from build123d import *

# Parameters (mm, degrees)
CORNER_DEPTH = 6
SKETCH2_W    = 6
SKETCH2_H    = 70
SKETCH2_H_2  = 260
MOUNT_DEPTH  = 10
FILLET1_R    = 1
LITE_DEPTH   = 391.911754748


with BuildPart() as part:
    # Sketch1 → corner (new body)
    with BuildSketch(Plane(origin=(0, 0, 0), x_dir=(0, 0, -1), z_dir=(1, 0, 0))):
        Polygon((0, 0), (0, 370), (26, 370), (126, 20), (126, 0), align=None)
    extrude(amount=CORNER_DEPTH)

    # Sketch2 → mount (cut)
    with BuildSketch(Plane(origin=(6, 0, 0), x_dir=(0, 0, -1), z_dir=(1, 0, 0))):
        with Locations((3, 335)):
            Rectangle(SKETCH2_W, SKETCH2_H)
        with Locations((3, 130)):
            Rectangle(SKETCH2_W, SKETCH2_H_2)
    extrude(amount=-MOUNT_DEPTH, mode=Mode.SUBTRACT)

    # Fillet1
    fillet1_edges = [part.edges().sort_by_distance(p)[0] for p in [
        (3, 370, -6),
        (3, 300, 0),
        (3, 260, 0),
        (3, 0, -6),
        (3, 370, -26),
        (3, 20, -126),
        (3, 0, -126),
    ]]
    fillet(fillet1_edges, radius=FILLET1_R)

    # Sketch3 → lite (cut, through all)
    with BuildSketch(Plane(origin=(6, 0, 0), x_dir=(0, 0, -1), z_dir=(1, 0, 0))):
        with BuildLine():
            Line((26.065623551, 228.856249777), (48.614841214, 32.99843711))
            ThreePointArc((48.614841214, 32.99843711), (68.661000724, 17.703495291), (83.182846647, 38.316591792))
            Line((83.182846647, 38.316591792), (45.818769512, 231.89519531))
            ThreePointArc((45.818769512, 231.89519531), (34.479428157, 239.883716977), (26.065623551, 228.856249777))
        make_face()
    extrude(amount=-LITE_DEPTH, mode=Mode.SUBTRACT)


solid = part.part
Read the model definition and answer for the solid it produces. Units are mm, in the model's axes. A direction names the side the tool comes from. Coordinates: 2 decimals unless noted, no trailing zeros. Loops run counter-clockwise (first coordinate to the right, second up) from the corner with the lowest first, then second, coordinate; pieces in that order, holes last.
Q1. The part is cut by section A-A on z = -62. Write down the section's boundary in (x, y), and give its area (3 significant figures).
Q2. Which of the six approach directions +Z, -Z, +X, -X, +Y, -Y give full straight-line access (tool end or side, diameter ignored) to faces 5 (the face through (3, 129, -6)), 6 (the face through (3, 11, -126)), 7 (the face through (3.042, 132.298, -37.182))?
Q3. The part is cut by section C-C on y = 102.5. Write down the section's boundary in (x, z).
Q4. Consider probe 1 along Z at (x, y) = (2.25, 158); probe 2 along Z at (x, y) = (4.5, 146.5); probe 3 along Z at (x, y) = (1.5, 295.5). Determine where each line is inside the solid, lowest interval first.
Q5. The part is cut by section B-B on x = 1. Write down the section's boundary in (y, z).
Q6. Each of these flat-tipped pins is pushed along its axis until it touches: pin 1 Ø1.5 at (x, z) = (1.5, -2.5) entering from -Y; pin 2 Ø1.8 at (x, y) = (1.5, 340.5) entering from +Z. Where does it stop, or does it pass through?
Q7. The part is cut by section D-D on z = -107.5. Write down the section's boundary in (x, y).
Q8. The mould has two halves that part along Y. Classify faces 1 (the face through (3, 197.1, -75.4)), 2 (the face through (3, 0, -67)), 3 (the face through (3.042, 239.914, -34.692)), 4 (the face through (3, 334, -6)): +Y half, -Y half, draft (parallel to the pull), parting line (faces both ways), or undercut.
Results below:
1. outline: (0, 0) - (6, 0) - (6, 17.96) - (0, 17.96) - close; (0, 148.06) - (6, 148.06) - (6, 244) - (0, 244) - close
1. area: 683 mm2
2. face 5: +Z, +X, -X, -Y
2. face 6: -Z, +X, -X, +Y, -Y
2. face 7: +X, -X
3. outline: (0, -102.43) - (6, -102.43) - (6, -70.79) - (0, -70.79) - close; (0, -40.61) - (6, -40.61) - (6, -6) - (0, -6) - close
4. probe 1: z = -86.57 to -60.08, -34.22 to -6
4. probe 2: z = -89.86 to -62.3, -35.55 to -6
4. probe 3: z = -47.29 to 0
5. outline: (0, -125) arc R1 ccw to (1, -126) - (19.86, -126) arc R1 ccw to (20.13, -125.96) - (369.27, -26.21) arc R1 ccw to (370, -25.25) - (370, -7) arc R1 ccw to (369, -6) - (300, -6) - (300, -1) arc R1 ccw to (299, 0) - (261, 0) arc R1 ccw to (260, -1) - (260, -6) - (1, -6) arc R1 ccw to (0, -7) - close; hole (33, -48.61) arc R17.5 ccw (long way) to (38.32, -83.18) - (231.9, -45.82) arc R10 ccw to (228.86, -26.07) - close
6. pin 1: stops at y = 260
6. pin 2: stops at z = -6
7. outline: (0, 0) - (6, 0) - (6, 84.75) - (0, 84.75) - close
8. face 1: +Y half
8. face 2: -Y half
8. face 3: undercut
8. face 4: draft
